CAD build for the part. Positions are in the model's coordinates, mm. Round coordinates to 2 decimals unless told otherwise and drop trailing zeros. Loops run counter-clockwise (first coordinate to the right, second up) from the corner with the lowest first, then second, coordinate; pieces in that order, holes last. Notation, with made-up numbers: M 3,89 L 37,89 A29 cw 37,118 Z; hole C -9,79 d6. An arc over 180 degrees is marked long. Put each result on its own line as item: value. Start each with the question number.
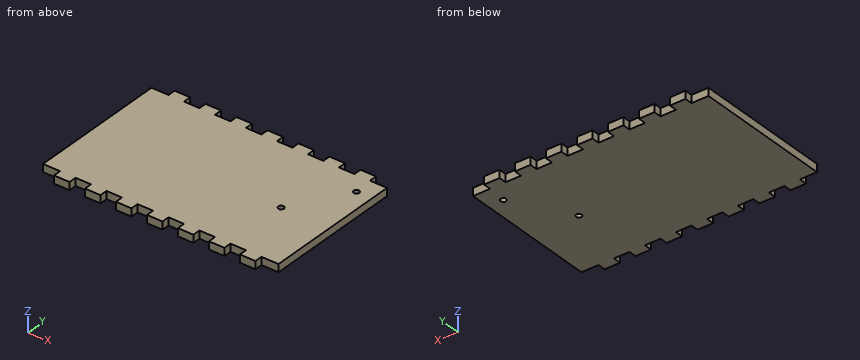
from build123d import *

# Parameters (mm, degrees)
SKETCH1_W           = 96.52
SKETCH1_H           = 63.5
BOSS_EXTRUDE1_DEPTH = 3.175
SKETCH2_W           = 6.985
SKETCH2_H           = 3.175
SKETCH2_W_2         = 6.35
CUT_EXTRUDE1_DEPTH  = 4.175
SKETCH3_R           = 1.143
CUT_EXTRUDE2_DEPTH  = 4.175


with BuildPart() as part:
    # Sketch1 → Boss-Extrude1 (new body)
    with BuildSketch(Plane.XY):
        Rectangle(SKETCH1_W, SKETCH1_H)
    extrude(amount=BOSS_EXTRUDE1_DEPTH)

    # Sketch2 → Cut-Extrude1 (cut, through all)
    with BuildSketch(Plane.XY.offset(3.175)):
        with Locations((-44.7675, -30.1625)):
            Rectangle(SKETCH2_W, SKETCH2_H)
        with Locations((-31.75, -30.1625)):
            Rectangle(SKETCH2_W_2, SKETCH2_H)
        with Locations((-19.05, -30.1625)):
            Rectangle(SKETCH2_W_2, SKETCH2_H)
        with Locations((-6.35, -30.1625)):
            Rectangle(SKETCH2_W_2, SKETCH2_H)
        with Locations((6.35, -30.1625)):
            Rectangle(SKETCH2_W_2, SKETCH2_H)
        with Locations((19.05, -30.1625)):
            Rectangle(SKETCH2_W_2, SKETCH2_H)
        with Locations((31.75, -30.1625)):
            Rectangle(SKETCH2_W_2, SKETCH2_H)
        with Locations((44.7675, -30.1625)):
            Rectangle(SKETCH2_W, SKETCH2_H)
        with Locations((44.7675, 30.1625)):
            Rectangle(SKETCH2_W, SKETCH2_H)
        with Locations((31.75, 30.1625)):
            Rectangle(SKETCH2_W_2, SKETCH2_H)
        with Locations((19.05, 30.1625)):
            Rectangle(SKETCH2_W_2, SKETCH2_H)
        with Locations((6.35, 30.1625)):
            Rectangle(SKETCH2_W_2, SKETCH2_H)
        with Locations((-6.35, 30.1625)):
            Rectangle(SKETCH2_W_2, SKETCH2_H)
        with Locations((-19.05, 30.1625)):
            Rectangle(SKETCH2_W_2, SKETCH2_H)
        with Locations((-31.75, 30.1625)):
            Rectangle(SKETCH2_W_2, SKETCH2_H)
        with Locations((-44.7675, 30.1625)):
            Rectangle(SKETCH2_W, SKETCH2_H)
    extrude(amount=-CUT_EXTRUDE1_DEPTH, mode=Mode.SUBTRACT)

    # Sketch3 → Cut-Extrude2 (cut, through all)
    with BuildSketch(Plane.XY.offset(3.175)):
        with Locations((28.3591, -1.6383)):
            Circle(SKETCH3_R)
        with Locations((41.91, 20.6883)):
            Circle(SKETCH3_R)
    extrude(amount=-CUT_EXTRUDE2_DEPTH, mode=Mode.SUBTRACT)


solid = part.part
(1) Cut at A-A on x = -20.5. List the corners of the cut face in (y, z) (3 decimals), and give its area (3 significant figures).
(2) Flat gauge pins, fed straight in: pin 1 Ø1 at (x, z) = (-31, 1.5) entering from +Y (3 decimals); pin 2 Ø1 at (y, z) = (30.5, 2.5) entering from +X (3 decimals); pin 3 Ø1.6 at (y, z) = (30.5, 1) entering from -X (3 decimals). Where does each tip first touch, or does it go through?
(3) Drill centre lines: line 1 along Y through (x, z) = (41.91, 2) (3 decimals); line 2 along Y through (x, z) = (-22, 2.5) (3 decimals); line 3 along Y through (x, z) = (29, 2.95) (3 decimals). Where is each one in solid material? Low to high.
(4) Cut at B-B on z = 1.85. Count the separate pieces of the cut face and the enclosed holes in it, and give its area (3 significant figures).
Taken from the geometry:
1. outline: M -28.575,0 L 28.575,0 L 28.575,3.175 L -28.575,3.175 Z
1. area: 181 mm2
2. pin 1: y = 28.575
2. pin 2: x = 41.275
2. pin 3: x = -41.275
3. line 1: -28.575 to 19.545, 21.831 to 28.575
3. line 2: -28.575 to 28.575
3. line 3: -28.575 to -2.585, -0.692 to 28.575
4. separate pieces: 1
4. enclosed holes: 2
4. area: 5,790 mm2
